```python
from build123d import *

# Parameters (mm, degrees)
EXTRUDE_1_DEPTH     = 265
SKETCH_2_R          = 1
CUT_EXTRUDE_1_DEPTH = 10
CHAMFER_1_SIZE      = 0.5
SKETCH_3_R          = 2.383304988
CUT_EXTRUDE_2_DEPTH = 1


with BuildPart() as part:
    # 草图1 → 凸台-拉伸1 (new body)
    with BuildSketch(Plane(origin=(0, 0, 0), x_dir=(1, 0, 0), z_dir=(0, 1, 0))):
        Polygon((-3.5, 0.4), (-3.5, -2.4), (3.5, -2.4), (3.5, 0.4), (2.5, 0.4), (2.5, 1.4), (3.5, 1.4), (3.5, 2.4), (-3.5, 2.4), (-3.5, 1.4), (-2.5, 1.4), (-2.5, 0.4), align=None)
    extrude(amount=EXTRUDE_1_DEPTH)

    # 草图2 → 切除-拉伸1 (cut)
    with BuildSketch(Plane(origin=(0, 0, -2.4), x_dir=(-1, 0, 0), z_dir=(0, 0, -1))):
        with Locations((0, 5)):
            Circle(SKETCH_2_R)
        with Locations((0, 20)):
            Circle(SKETCH_2_R)
        with Locations((0, 35)):
            Circle(SKETCH_2_R)
        with Locations((0, 50)):
            Circle(SKETCH_2_R)
        with Locations((0, 65)):
            Circle(SKETCH_2_R)
        with Locations((0, 80)):
            Circle(SKETCH_2_R)
        with Locations((0, 95)):
            Circle(SKETCH_2_R)
        with Locations((0, 110)):
            Circle(SKETCH_2_R)
        with Locations((0, 125)):
            Circle(SKETCH_2_R)
        with Locations((0, 140)):
            Circle(SKETCH_2_R)
        with Locations((0, 155)):
            Circle(SKETCH_2_R)
        with Locations((0, 170)):
            Circle(SKETCH_2_R)
        with Locations((0, 185)):
            Circle(SKETCH_2_R)
        with Locations((0, 200)):
            Circle(SKETCH_2_R)
        with Locations((0, 215)):
            Circle(SKETCH_2_R)
        with Locations((0, 230)):
            Circle(SKETCH_2_R)
        with Locations((0, 245)):
            Circle(SKETCH_2_R)
        with Locations((0, 260)):
            Circle(SKETCH_2_R)
    extrude(amount=-CUT_EXTRUDE_1_DEPTH, mode=Mode.SUBTRACT)

    # 倒角1
    chamfer_1_edges = [part.edges().sort_by_distance(p)[0] for p in [
        (-3.5, 132.5, -2.4),
        (3.5, 132.5, -2.4),
        (3.5, 132.5, 2.4),
        (-3.5, 132.5, 2.4),
    ]]
    chamfer(chamfer_1_edges, length=CHAMFER_1_SIZE)

    # 草图3 → 切除-拉伸2 (cut)
    with BuildSketch(Plane(origin=(0, 0, -2.4), x_dir=(-1, 0, 0), z_dir=(0, 0, -1))):
        with Locations((0, 5)):
            Circle(SKETCH_3_R)
        with Locations((0, 20)):
            Circle(SKETCH_3_R)
        with Locations((0, 35)):
            Circle(SKETCH_3_R)
        with Locations((0, 50)):
            Circle(SKETCH_3_R)
        with Locations((0, 65)):
            Circle(SKETCH_3_R)
        with Locations((0, 80)):
            Circle(SKETCH_3_R)
        with Locations((0, 95)):
            Circle(SKETCH_3_R)
        with Locations((0, 110)):
            Circle(SKETCH_3_R)
        with Locations((0, 125)):
            Circle(SKETCH_3_R)
        with Locations((0, 140)):
            Circle(SKETCH_3_R)
        with Locations((0, 155)):
            Circle(SKETCH_3_R)
        with Locations((0, 170)):
            Circle(SKETCH_3_R)
        with Locations((0, 185)):
            Circle(SKETCH_3_R)
        with Locations((0, 200)):
            Circle(SKETCH_3_R)
        with Locations((0, 215)):
            Circle(SKETCH_3_R)
        with Locations((0, 230)):
            Circle(SKETCH_3_R)
        with Locations((0, 245)):
            Circle(SKETCH_3_R)
        with Locations((0, 260)):
            Circle(SKETCH_3_R)
    extrude(amount=-CUT_EXTRUDE_2_DEPTH, mode=Mode.SUBTRACT)


solid = part.part
```
The model under review builds one solid part; all positions refer to its coordinate system, in mm. A direction names the side the tool comes from. Round coordinates to 2 decimals unless told otherwise and drop trailing zeros. Loops run counter-clockwise (first coordinate to the right, second up) from the corner with the lowest first, then second, coordinate; pieces in that order, holes last. Notation, with made-up numbers: (-20, 29.25) - (29, 29.25) arc R19 ccw to (29, 64.25) - close; hole circle Ø8 at (27.5, -37). An arc over 180 degrees is marked (long way). Write each question's results on one line, items separated by ' | '. Start each with the question number.
Q1. Tool access review of faces 4 (the flat face through (0, 131, -2.4)), 5 (the cylindrical face through (0.517, 92.673, -1.907)): name each direction out of +Z, -Z, +X, -X, +Y, -Y from which nothing blocks a thin tool from reaching the whole face with its end or side.
Q2. Draft analysis for pull direction Y (two halves, no side actions). For faces 1 (the cylindrical face through (-1.1, 47.886, -1.907)), 2 (the flat face through (0, 131, 2.4)), 3 (the flat face through (0, 265, 0)), state which applies: pulls with the +Y half, pulls with the -Y half, needs draft (parallel to the pull), parting line crosses it, or undercut.
Q3. Wall thickness on line 1 along Z through (x, y) = (2.75, 243); line 2 along X through (y, z) = (170, -1.95); line 3 along X through (y, z) = (27, -1.25): over which ranges is each line inside the solid? List them lowest first. Write a range as [from, to].
Q4. Take a section at A-A on z = 0.6. Give the number of separate pieces and of enclosed holes in the cut face, plus the area to 3 significant figures.
Q5. Take a section at B-B on y = 160. Give the boundary of the cut face in (x, z), plus the area to 3 significant figures.
Q6. Insertion check: P1, Ø1.2, axis at x = 0, y = 20, coming from the -Z side; P2, Ø4, axis at x = 0, y = 125, coming from the -Z side. Each pin has a flat end and moves straight along its axis. Give the tip position at first contact, or say it passes through.
Data:
1) face 4: -Z, +X, -X, +Y, -Y | face 5: -Z
2) face 1: undercut | face 2: needs draft | face 3: pulls with the +Y half
3) line 1: z = [-2.4, -1.4], [-0.4, 2.4] | line 2: x = [-3.45, -2.38], [2.38, 3.45] | line 3: x = [-2.5, 2.5]
4) separate pieces: 1 | enclosed holes: 18 | area: 1,800 mm²
5) outline: (-3.5, -1.9) - (-3, -2.4) - (3, -2.4) - (3.5, -1.9) - (3.5, -1.4) - (2.5, -1.4) - (2.5, -0.4) - (3.5, -0.4) - (3.5, 1.9) - (3, 2.4) - (-3, 2.4) - (-3.5, 1.9) - (-3.5, -0.4) - (-2.5, -0.4) - (-2.5, -1.4) - (-3.5, -1.4) - close | area: 31.1 mm²
6) P1: passes through | P2: stops at z = -1.4
